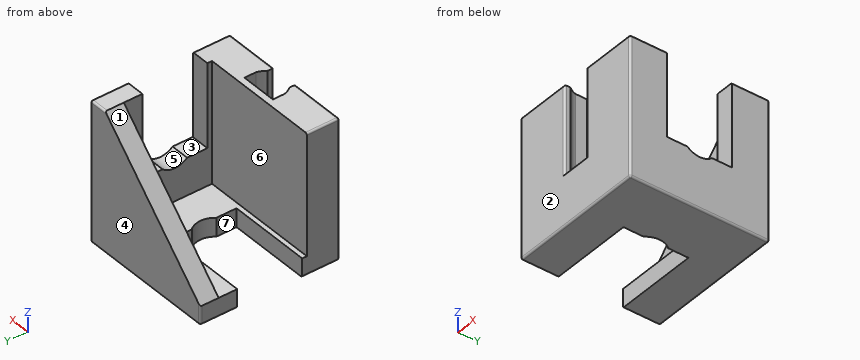
from build123d import *

# Parameters (mm, degrees)
SKETCH_1_W                      = 15
SKETCH_1_H                      = 15
EXTRUDE_1_DEPTH                 = 15
SKETCH_2_W                      = 13
SKETCH_2_H                      = 9.5
CUT_EXTRUDE_1_DEPTH             = 13
CUT_EXTRUDE_2_DEPTH             = 9.45
EXTRUDE_START                   = -4.5
EXTRUDE_2_DEPTH                 = 6
SKETCH_5_W                      = 3
SKETCH_5_H                      = 3
EXTRUDE_3_DEPTH                 = 1
CUT_EXTRUDE_3_REACH             = 26.238
CUT_EXTRUDE_4_REACH             = 29.5
CUT_EXTRUDE_5_REACH             = 26.238
CUT_EXTRUDE_5_DIRECTION_2_REACH = 26.238
SKETCH_10_W                     = 5.767295788
SKETCH_10_H                     = 2.858107371
CUT_EXTRUDE_7_DEPTH             = 25.238399287
CUT_EXTRUDE_8_DEPTH             = 2
FILLET_2_R                      = 0.2
CUT_EXTRUDE_9_REACH             = 26.88
SKETCH_12_W                     = 9
SKETCH_12_H                     = 7
CUT_EXTRUDE_10_REACH            = 23.219
SKETCH_13_W                     = 9
SKETCH_13_H                     = 7


with BuildPart() as part:
    # Sketch 1 → Extrude 1 (new body)
    with BuildSketch(Plane.XY):
        with Locations((0, 7.5)):
            Rectangle(SKETCH_1_W, SKETCH_1_H)
    extrude(amount=-EXTRUDE_1_DEPTH)

    # Sketch 2 → Cut-Extrude 1 (cut)
    with BuildSketch(Plane.ZY.offset(7.5)):
        with Locations((-6.5, 8.25)):
            Rectangle(SKETCH_2_W, SKETCH_2_H)
    extrude(amount=-CUT_EXTRUDE_1_DEPTH, mode=Mode.SUBTRACT)

    # Sketch 3 → Cut-Extrude 2 (cut)
    with BuildSketch(Plane.XY):
        with BuildLine():
            Line((-1.5, 0), (-1.5, 0.677124344))
            ThreePointArc((-1.5, 0.677124344), (-1.780042303, 1.088161527), (-1.95, 1.555590279))
            Line((-1.95, 1.555590279), (-1.95, 2.8))
            Line((-1.95, 2.8), (1.95, 2.8))
            Line((1.95, 2.8), (1.95, 1.555590279))
            ThreePointArc((1.95, 1.555590279), (1.780042303, 1.088161527), (1.5, 0.677124344))
            Line((1.5, 0.677124344), (1.5, 0))
            Line((1.5, 0), (-1.5, 0))
        make_face()
    extrude(amount=-CUT_EXTRUDE_2_DEPTH, mode=Mode.SUBTRACT)



with BuildPart() as body_2:
    # Sketch 4 → Extrude 2 (new body)
    with BuildSketch(Plane.XY.offset(EXTRUDE_START)):
        with BuildLine():
            Line((-1.5, 15.677124344), (1.5, 15.677124344))
            ThreePointArc((1.5, 15.677124344), (1.780042303, 16.088161527), (1.95, 16.555590279))
            Line((1.95, 16.555590279), (1.95, 17.5))
            Line((1.95, 17.5), (-1.95, 17.5))
            Line((-1.95, 17.5), (-1.95, 16.555590279))
            ThreePointArc((-1.95, 16.555590279), (-1.780042303, 16.088161527), (-1.5, 15.677124344))
        make_face()
    extrude(amount=-EXTRUDE_2_DEPTH)


with BuildPart() as part_1:
    add(part.part)

    add(body_2.part)  # Extrude 3 merges body 2
    # Sketch 5 → Extrude 3 (add)
    with BuildSketch(Plane(origin=(0, 15, 0), x_dir=(-1, 0, 0), z_dir=(0, 1, 0))):
        with Locations((0, -7.5)):
            Rectangle(SKETCH_5_W, SKETCH_5_H)
    extrude(amount=EXTRUDE_3_DEPTH)

    # Sketch 6 → Cut-Extrude 3 (cut, up to next)
    with BuildSketch(Plane(origin=(0, 0, -15), x_dir=(-1, 0, 0), z_dir=(0, 0, -1)), mode=Mode.PRIVATE) as cut_extrude_3_sk1:
        with BuildLine():
            Line((-1.5, 6.177124344), (-1.5, 4))
            Line((-1.5, 4), (1.5, 4))
            Line((1.5, 4), (1.5, 6.177124344))
            ThreePointArc((1.5, 6.177124344), (2, 7.5), (1.5, 8.822875656))
            Line((1.5, 8.822875656), (1.5, 11))
            Line((1.5, 11), (-1.5, 11))
            Line((-1.5, 11), (-1.5, 8.822875656))
            ThreePointArc((-1.5, 8.822875656), (-2, 7.5), (-1.5, 6.177124344))
        make_face()
    cut_extrude_3_tool1 = extrude(cut_extrude_3_sk1.sketch, amount=-CUT_EXTRUDE_3_REACH, mode=Mode.PRIVATE) & part_1.part
    add(cut_extrude_3_tool1.solids().sort_by_distance((0, 7.5, -15))[0], mode=Mode.SUBTRACT)

    # Sketch 7 → Cut-Extrude 4 (cut, up to next)
    with BuildSketch(Plane(origin=(7.5, 0, 0), x_dir=(0, 0, -1), z_dir=(1, 0, 0)), mode=Mode.PRIVATE) as cut_extrude_4_sk1:
        with BuildLine():
            Line((6, 6.177124344), (6, 4))
            Line((6, 4), (9, 4))
            Line((9, 4), (9, 6.177124344))
            ThreePointArc((9, 6.177124344), (9.5, 7.5), (9, 8.822875656))
            Line((9, 8.822875656), (9, 11))
            Line((9, 11), (6, 11))
            Line((6, 11), (6, 8.822875656))
            ThreePointArc((6, 8.822875656), (5.5, 7.5), (6, 6.177124344))
        make_face()
    cut_extrude_4_tool1 = extrude(cut_extrude_4_sk1.sketch, amount=-CUT_EXTRUDE_4_REACH, mode=Mode.PRIVATE) & part_1.part
    add(cut_extrude_4_tool1.solids().sort_by_distance((7.5, 7.5, -7.5))[0], mode=Mode.SUBTRACT)

    # Sketch 8 → Cut-Extrude 5 (cut, up to next)
    with BuildSketch(Plane(origin=(0, 0, 0), x_dir=(0, 0, -1), z_dir=(1, 0, 0)), mode=Mode.PRIVATE) as cut_extrude_5_sk1:
        with BuildLine():
            Line((5.55, 17.5), (5.55, 16.555590279))
            ThreePointArc((5.55, 16.555590279), (5.719957697, 16.088161527), (6, 15.677124344))
            Line((6, 15.677124344), (4.5, 15.677124344))
            Line((4.5, 15.677124344), (4.5, 17.5))
            Line((4.5, 17.5), (5.55, 17.5))
        make_face()
    cut_extrude_5_tool1 = extrude(cut_extrude_5_sk1.sketch, amount=-CUT_EXTRUDE_5_REACH, mode=Mode.PRIVATE) & part_1.part
    # Sketch 8 → Cut-Extrude 5 (cut, up to next)
    with BuildSketch(Plane(origin=(0, 0, 0), x_dir=(0, 0, -1), z_dir=(1, 0, 0)), mode=Mode.PRIVATE) as cut_extrude_5_sk2:
        with BuildLine():
            Line((10.5, 17.5), (9.45, 17.5))
            Line((9.45, 17.5), (9.45, 16.555590279))
            ThreePointArc((9.45, 16.555590279), (9.280042303, 16.088161527), (9, 15.677124344))
            Line((9, 15.677124344), (10.5, 15.677124344))
            Line((10.5, 15.677124344), (10.5, 17.5))
        make_face()
    cut_extrude_5_tool2 = extrude(cut_extrude_5_sk2.sketch, amount=-CUT_EXTRUDE_5_REACH, mode=Mode.PRIVATE) & part_1.part
    add(cut_extrude_5_tool1.solids().sort_by_distance((0, 16.539049, -5.075076))[0], mode=Mode.SUBTRACT)
    add(cut_extrude_5_tool2.solids().sort_by_distance((0, 16.539049, -9.924924))[0], mode=Mode.SUBTRACT)

    # Sketch 8 → Cut-Extrude 5 direction 2 (cut, up to next)
    with BuildSketch(Plane(origin=(0, 0, 0), x_dir=(0, 0, -1), z_dir=(1, 0, 0)), mode=Mode.PRIVATE) as cut_extrude_5_direction_2_sk1:
        with BuildLine():
            Line((5.55, 17.5), (5.55, 16.555590279))
            ThreePointArc((5.55, 16.555590279), (5.719957697, 16.088161527), (6, 15.677124344))
            Line((6, 15.677124344), (4.5, 15.677124344))
            Line((4.5, 15.677124344), (4.5, 17.5))
            Line((4.5, 17.5), (5.55, 17.5))
        make_face()
    cut_extrude_5_direction_2_tool1 = extrude(cut_extrude_5_direction_2_sk1.sketch, amount=CUT_EXTRUDE_5_DIRECTION_2_REACH, mode=Mode.PRIVATE) & part_1.part
    # Sketch 8 → Cut-Extrude 5 direction 2 (cut, up to next)
    with BuildSketch(Plane(origin=(0, 0, 0), x_dir=(0, 0, -1), z_dir=(1, 0, 0)), mode=Mode.PRIVATE) as cut_extrude_5_direction_2_sk2:
        with BuildLine():
            Line((10.5, 17.5), (9.45, 17.5))
            Line((9.45, 17.5), (9.45, 16.555590279))
            ThreePointArc((9.45, 16.555590279), (9.280042303, 16.088161527), (9, 15.677124344))
            Line((9, 15.677124344), (10.5, 15.677124344))
            Line((10.5, 15.677124344), (10.5, 17.5))
        make_face()
    cut_extrude_5_direction_2_tool2 = extrude(cut_extrude_5_direction_2_sk2.sketch, amount=CUT_EXTRUDE_5_DIRECTION_2_REACH, mode=Mode.PRIVATE) & part_1.part
    add(cut_extrude_5_direction_2_tool1.solids().sort_by_distance((0, 16.539049, -5.075076))[0], mode=Mode.SUBTRACT)
    add(cut_extrude_5_direction_2_tool2.solids().sort_by_distance((0, 16.539049, -9.924924))[0], mode=Mode.SUBTRACT)

    # Sketch 10 → Cut-Extrude 7 (cut, through all)
    with BuildSketch(Plane.XY):
        with Locations((0, 16.429053686)):
            Rectangle(SKETCH_10_W, SKETCH_10_H)
    extrude(amount=-CUT_EXTRUDE_7_DEPTH, mode=Mode.SUBTRACT)

    # Sketch 11 → Cut-Extrude 8 (cut)
    with BuildSketch(Plane(origin=(0, 15, 0), x_dir=(-1, 0, 0), z_dir=(0, 1, 0))):
        Polygon((7.5, -13), (7.5, 0), (-5.5, 0), align=None)
    extrude(amount=-CUT_EXTRUDE_8_DEPTH, mode=Mode.SUBTRACT)

    # Fillet 2
    fillet_2_edges = [part_1.edges().sort_by_distance(p)[0] for p in [
        (7.5, 7.5, -15),
        (0, 15, -15),
        (-7.5, 1.75, 0),
        (4.5, 0, 0),
        (0, 0, -9.45),
        (1.5, 0, -4.725),
        (-1.5, 0, -4.725),
        (-7.5, 7.5, -15),
        (6.5, 15, 0),
        (7.5, 7.5, 0),
        (-4.5, 0, 0),
        (0, 0, -15),
        (-7.5, 15, -14),
        (7.5, 15, -7.5),
        (7.5, 0, -7.5),
        (-7.5, 0, -7.5),
    ]]
    fillet(fillet_2_edges, radius=FILLET_2_R)

    # Sketch 12 → Cut-Extrude 9 (cut, up to next)
    with BuildSketch(Plane.ZY.offset(-5.5), mode=Mode.PRIVATE) as cut_extrude_9_sk1:
        with Locations((-4.5, 7.5)):
            Rectangle(SKETCH_12_W, SKETCH_12_H)
    cut_extrude_9_tool1 = extrude(cut_extrude_9_sk1.sketch, amount=-CUT_EXTRUDE_9_REACH, mode=Mode.PRIVATE) & part_1.part
    add(cut_extrude_9_tool1.solids().sort_by_distance((5.5, 7.5, -4.5))[0], mode=Mode.SUBTRACT)

    # Sketch 13 → Cut-Extrude 10 (cut, up to next)
    with BuildSketch(Plane.XY.offset(-13), mode=Mode.PRIVATE) as cut_extrude_10_sk1:
        with Locations((-3, 7.5)):
            Rectangle(SKETCH_13_W, SKETCH_13_H)
    cut_extrude_10_tool1 = extrude(cut_extrude_10_sk1.sketch, amount=-CUT_EXTRUDE_10_REACH, mode=Mode.PRIVATE) & part_1.part
    add(cut_extrude_10_tool1.solids().sort_by_distance((-3, 7.5, -13))[0], mode=Mode.SUBTRACT)


solid = part_1.part
Geometry: final body of the model. Coordinates: model frame, mm. Face numbers are marked on the shaded views. A direction names the side the tool comes from. Coordinates: 2 decimals unless noted, no trailing zeros. Order: outer loops, then holes, each group sorted by start corner. A loop starts at its lowest first (then second) coordinate and runs counter-clockwise, first axis right, second up.
(1) Access query for the marked faces 5, 6 and 7. Directions: +Z, -Z, +X, -X, +Y, -Y. A direction counts if a zero-diameter tool reaches every point of the face in a straight line with its end or side. Return the directions, or none.
(2) Section query C-C (y = 10). Return the cut outline in (x, z), plus the area to 3 significant figures.
(3) Material intervals for probe 1 along X at (y, z) = (2, -2); probe 2 along Y at (x, z) = (3.25, -2.5); probe 3 along Y at (x, z) = (-5.5, -4.5), sorted ascending.
(4) Draft query along Y for the marked faces 1, 2, 3 and 4. Return one class per face: pulls with the +Y half, pulls with the -Y half, needs draft (parallel to the pull), parting line crosses it, or undercut.
(5) Section query B-B (x = -6.25). Return the cut outline in (y, z), plus the area to 3 significant figures.
(6) Section query A-A (z = -2). Return the cut outline in (x, y).
(7) First-contact query: pin 1 (7.5 mm diameter, centred on y = 8, z = -3.5, fed in from -X); pin 2 (1.6 mm diameter, centred on y = 9.5, z = -14.5, fed in from -X). Flat tips, straight axial feed; report the tip coordinate or a pass-through.
(8) Section query D-D (x = 3.75). Return the cut outline in (y, z).
Solution:
1. face 5: +Z, +X, -X
1. face 6: +Z, -X
1. face 7: +Z, -Z, -X
2. outline: (1.5, -15) - (7.3, -15) arc R0.2 ccw to (7.5, -14.8) - (7.5, -9) - (5.5, -9) - (5.5, -13) - (1.5, -13) - close
2. area: 20.0 mm2
3. probe 1: x = -7.5 to -1.95, 1.95 to 7.5
3. probe 2: y = 0 to 3.5, 13 to 15
3. probe 3: y = 0 to 3.5
4. face 1: needs draft
4. face 2: pulls with the -Y half
4. face 3: undercut
4. face 4: pulls with the +Y half
5. outline: (0, -14.8) arc R0.2 ccw to (0.2, -15) - (4, -15) - (4, -13) - (3.5, -13) - (3.5, 0) - (0.2, 0) arc R0.2 ccw to (0, -0.2) - close; (11, -15) - (14.8, -15) arc R0.2 ccw to (15, -14.8) - (15, -11.75) - (13, -11.75) - (13, -13) - (11, -13) - close
5. area: 64.0 mm2
6. outline: (-7.5, 0.2) arc R0.2 ccw to (-7.3, 0) - (-1.7, 0) arc R0.2 ccw to (-1.5, 0.2) - (-1.5, 0.68) arc R2 cw to (-1.95, 1.56) - (-1.95, 2.8) - (1.95, 2.8) - (1.95, 1.56) arc R2 cw to (1.5, 0.68) - (1.5, 0.2) arc R0.2 ccw to (1.7, 0) - (7.3, 0) arc R0.2 ccw to (7.5, 0.2) - (7.5, 4) - (5.5, 4) - (5.5, 3.5) - (-7.5, 3.5) - close; (3.5, 13) - (5.5, 13) - (5.5, 11) - (7.5, 11) - (7.5, 14.8) arc R0.2 ccw to (7.3, 15) - (3.5, 15) - close
7. pin 1: stops at x = 5.5
7. pin 2: stops at x = 1.5
8. outline: (0, -14.8) arc R0.2 ccw to (0.2, -15) - (14.8, -15) arc R0.2 ccw to (15, -14.8) - (15, -1.75) - (13, -1.75) - (13, -13) - (3.5, -13) - (3.5, 0) - (0.2, 0) arc R0.2 ccw to (0, -0.2) - close
